Design review of the part shown in the three views and the two pictorial views. Dimensions are in mm from the part's minimum x, y and z. A direction names the side the tool comes from. Give positions to 0.01 mm unless a question says otherwise; leave off trailing zeros. Loops run counter-clockwise (first coordinate to the right, second up) from the corner with the lowest first, then second, coordinate; pieces in that order, holes last. Notation, with made-up numbers: (26, 41.5) -> (85, 41.5) arc R20 cw to (85, 54.5) -> close; hole circle Ø11 at (42, 23). An arc over 180 degrees is marked (long way). One line per question, with ' | ' between items. Start each with the question number.
(1) Wall thickness on probe 1 along Y at (x, z) = (95, 17); probe 2 along X at (y, z) = (96, 45); probe 3 along Z at (x, y) = (101.5, 31): over which ranges is each line inside the solid? List them lowest first.
(2) Consider section A-A (y = 95). Write out the cut boundary in (x, z).
(3) Consider section C-C (z = 30.5). Write out the cut boundary in (x, y), and give its area (3 significant figures).
(4) Insertion check: P1, Ø1, axis at x = 48, y = 78, coming from the -Z side; P2, Ø1.5, axis at y = 94.5, z = 52, coming from the -X side; P3, Ø4, axis at x = 74, z = 51.5, coming from the +Y side; P4, Ø1.5, axis at y = 76, z = 20.5, coming from the +X side. Each pin has a flat end and moves straight along its axis. Give the tip position at first contact, or say it passes through.
(5) Consider section D-D (y = 54.5). Write out the cut boundary in (x, z), and give its area (3 significant figures).
(6) Tool access review of the marked faces 1 and 2: name each direction out of +Z, -Z, +X, -X, +Y, -Y from which nothing blocks a thin tool from reaching the whole face with its end or side.
(7) Draft analysis for pull direction Z (two halves, no side actions). For the marked faces 3, 4 and 5, state which applies: +Z half, -Z half, draft (parallel to the pull), parting line (faces both ways), or undercut.
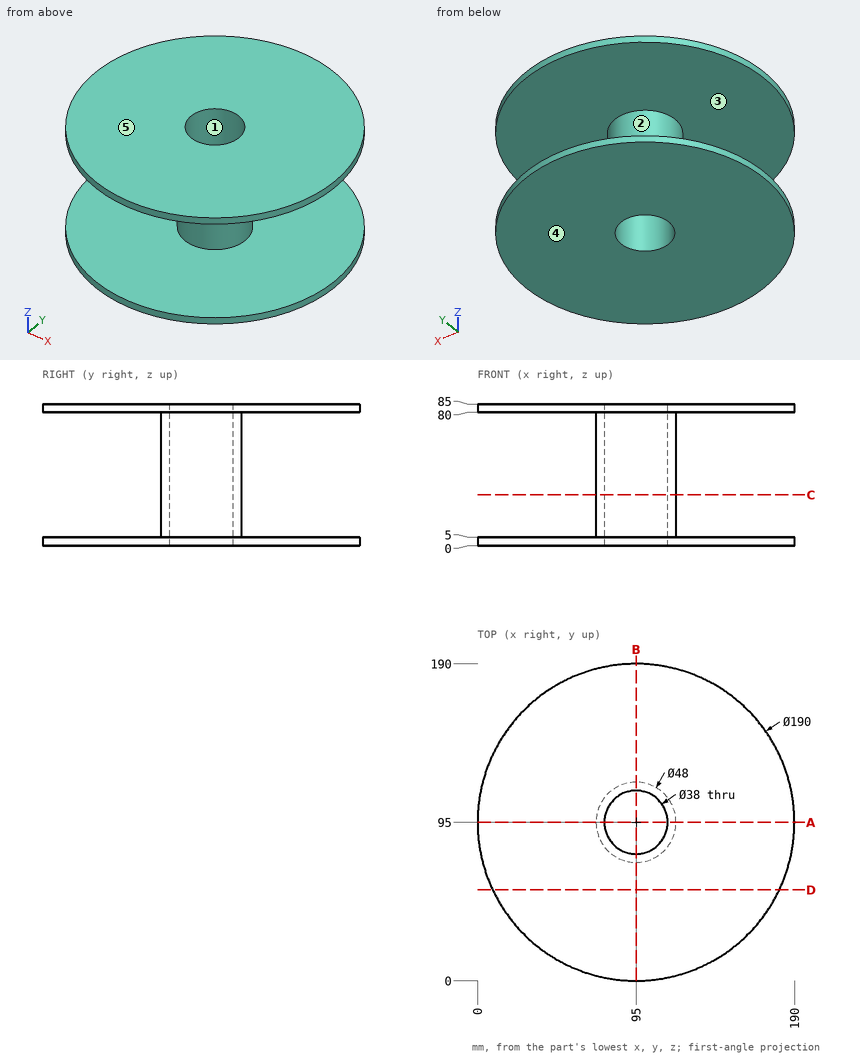
A:
1) probe 1: y = 71 to 76, 114 to 119 | probe 2: x = 71.02 to 76.03, 113.97 to 118.98 | probe 3: z = 0 to 5, 80 to 85
2) outline: (0, 0) -> (76, 0) -> (76, 85) -> (0, 85) -> (0, 80) -> (71, 80) -> (71, 5) -> (0, 5) -> close; (114, 0) -> (190, 0) -> (190, 5) -> (119, 5) -> (119, 80) -> (190, 80) -> (190, 85) -> (114, 85) -> close
3) outline: circle Ø48 at (95, 95); hole circle Ø38 at (95, 95) | area: 675 mm^2
4) P1: stops at z = 0 | P2: stops at x = 71 | P3: stops at y = 109.66 | P4: stops at x = 110.59
5) outline: (9.07, 0) -> (180.93, 0) -> (180.93, 5) -> (9.07, 5) -> close; (9.07, 80) -> (180.93, 80) -> (180.93, 85) -> (9.07, 85) -> close | area: 1,720 mm^2
6) face 1: +Z, -Z | face 2: none
7) face 3: undercut | face 4: -Z half | face 5: +Z half
